The figure shows three views and two pictorial views of one solid part (mm, origin at its lowest corner). Answer the questions. Give positions to 0.01 mm unless a question says otherwise; leave off trailing zeros. Write each loop counter-clockwise with the first axis right and the second up, starting at its lowest first coordinate (ties: lowest second). Pieces come first, ordered by that corner, then holes. Notation, with made-up numbers: M 80.25,14 L 120.25,14 A17 ccw 120.25,24 Z; hole C 83.5,65 d5. An arc over 180 degrees is marked long. Return JSON: item names as keys, results as strings.
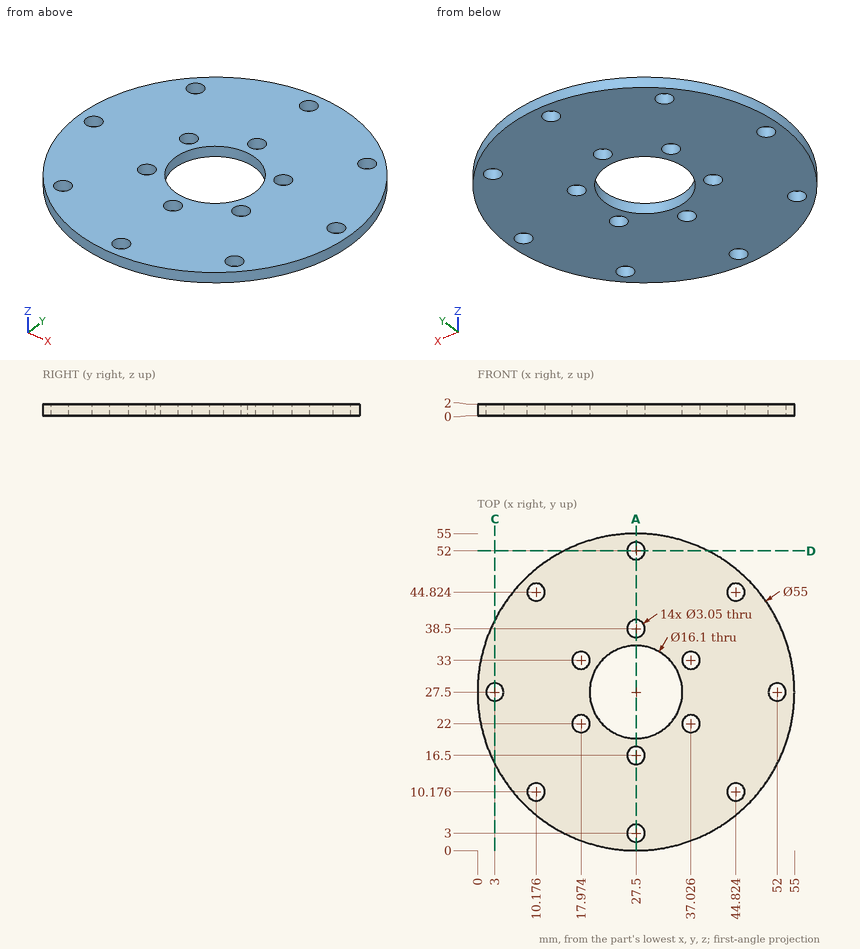
Item 1: Given pin 1 Ø1.8 at (x, y) = (3, 27.5) entering from +Z; pin 2 Ø3.5 at (x, y) = (44.82, 44.82) entering from +Z; pin 3 Ø1 at (x, z) = (41.5, 0.5) entering from +Y, each flat-ended and moving along its own axis, determine where each tip first touches the part or whether it passes through.
Geometry results:
{"pin 1": "passes through", "pin 2": "stops at z = 2", "pin 3": "stops at y = 51.46"}
Item 2: A cutting plane is placed at C-C, the plane x = 3. Write down the section's boundary in (y, z) (1 decimal).
Geometry results:
{"outline": "M 15,0 L 26,0 L 26,2 L 15,2 Z; M 29,0 L 40,0 L 40,2 L 29,2 Z"}
Item 3: Find the intervals of material crossed by line 1 (Y direction, x = 9, z = 0.5) (1 decimal); line 2 (X direction, y = 23, z = 1.05) (1 decimal); line 3 (Y direction, x = 32, z = 0.4) (1 decimal), in increasing order.
Geometry results:
{"line 1": "y = 7.2 to 9.2, 11.1 to 43.9, 45.8 to 47.8", "line 2": "x = 0.4 to 16.8, 19.1 to 20.8, 34.2 to 35.9, 38.2 to 54.6", "line 3": "y = 0.4 to 20.8, 34.2 to 54.6"}
Item 4: A cutting plane is placed at A-A, the plane x = 27.5. Count the separate pieces of the cut face and the enclosed holes in it, plus the area to 3 significant figures.
Geometry results:
{"separate pieces": "6", "enclosed holes": "0", "area": "53.4 mm2"}
